Source: CAD feature listing. Evaluate the final solid. Frame: model axes, mm. A direction names the side the tool comes from. Coordinates: 2 decimals unless noted, no trailing zeros. Order: outer loops, then holes, each group sorted by start corner. A loop starts at its lowest first (then second) coordinate and runs counter-clockwise, first axis right, second up.
```python
from build123d import *

# Parameters (mm, degrees)
F0_R     = 12.7
F1_DEPTH = 6.35
F2_R     = 3.175
F3_DEPTH = 25.4
F7_DEPTH = 3.175


with BuildPart() as f1:
    # F0 (on Top) → F1 (new body)
    with BuildSketch(Plane.XY):
        Circle(F0_R)
    extrude(amount=F1_DEPTH)

    # F2 (on face) → F3 (join)
    with BuildSketch(Plane(origin=(0, 0, 0), x_dir=(1, 0, 0), z_dir=(0, 0, -1))):
        Circle(F2_R)
    extrude(amount=F3_DEPTH)

    # F4 (on Right) → F5 (revolve)
    with BuildSketch(Plane.YZ):
        with BuildLine():
            Line((0, -28.575), (0, -25.4))
            Line((0, -25.4), (-3.175, -25.4))
            ThreePointArc((-3.175, -25.4), (-2.245064, -27.645064), (0, -28.575))
        make_face()
    revolve(axis=Axis((0, 0, -12.7), (0, 0, -1)))

    # F6 (on face) → F7 (join)
    with BuildSketch(Plane.XY.offset(6.35)):
        with BuildLine():
            Line((-10.16, -17.78), (0, -17.78))
            Line((0, -17.78), (10.16, -17.78))
            Line((10.16, -17.78), (19.05, 17.78))
            Line((19.05, 17.78), (20.244957, 22.55983))
            ThreePointArc((20.244957, 22.55983), (0, 25.2984), (-20.244957, 22.55983))
            Line((-20.244957, 22.55983), (-19.05, 17.78))
            Line((-19.05, 17.78), (-10.16, -17.78))
        make_face()
    extrude(amount=F7_DEPTH)


solid = f1.part
```
Q1. Section query B-B on x = 5. Output: boundary loops of the cut face in (y, z) (3 decimals), plus the area to 3 significant figures.
Solutions:
outline: (-17.78, 6.35) - (-11.674, 6.35) - (-11.674, 0) - (11.674, 0) - (11.674, 6.35) - (25.134, 6.35) - (25.134, 9.525) - (-17.78, 9.525) - close
area: 285 mm2
Q2. Material intervals for line 1 along Z through (x, y) = (-4.5, -11.5) (3 decimals); line 2 along Z through (x, y) = (-15.5, 19) (3 decimals); line 3 along X through (y, z) = (-0.5, -27), sorted ascending.
Solutions:
line 1: z = 0 to 9.525
line 2: z = 6.35 to 9.525
line 3: x = -2.7 to 2.7
Q3. Pin query (flat end, axial travel): P1, Ø7.5, axis at x = -4, y = -1, coming from the -Z side; P2, Ø12, axis at x = 8, y = 8, coming from the -Z side; P3, Ø12, axis at y = 9.5, z = -12.5, coming from the +X side; P4, Ø4, axis at x = -13.5, y = 14.5, coming from the -Z side. Return the tip coordinate at first contact, or that it passes through.
Solutions:
P1: stops at z = -28.55
P2: stops at z = 0
P3: passes through
P4: stops at z = 6.35
Q4. Set-up query: faces 1 (the flat face through (0, 4, 9.525)), 2 (the flat face through (0, 14, 6.35)). Return all of +Z, -Z, +X, -X, +Y, -Y with unobstructed straight access to the full face (end or side cutting, diameter ignored); none if empty.
Solutions:
face 1: +Z, +X, -X, +Y, -Y
face 2: -Z
Q5. Section query C-C on z = -3.5. Output: boundary loops of the cut face in (x, y) (3 decimals), plus the area to 3 significant figures.
Solutions:
outline: circle Ø6.35 at (0, 0)
area: 31.7 mm2
Q6. Section query A-A on y = 5.5. Output: boundary loops of the cut face in (x, z) (3 decimals).
Solutions:
outline: (-15.98, 6.35) - (-11.447, 6.35) - (-11.447, 0) - (11.447, 0) - (11.447, 6.35) - (15.98, 6.35) - (15.98, 9.525) - (-15.98, 9.525) - close
